Here's how the part is built. I have some questions about the finished solid (model axes, mm). Face numbers are marked on the shaded views. Give positions to 0.01 mm unless a question says otherwise; leave off trailing zeros. Write each loop counter-clockwise with the first axis right and the second up, starting at its lowest first coordinate (ties: lowest second). Pieces come first, ordered by that corner, then holes. Notation, with made-up numbers: (10, -24.5) -> (36, -24.5) arc R37 cw to (36, 11.5) -> close; hole circle Ø4 at (81, 33). An arc over 180 degrees is marked (long way). Use one line per item in the form item = value.
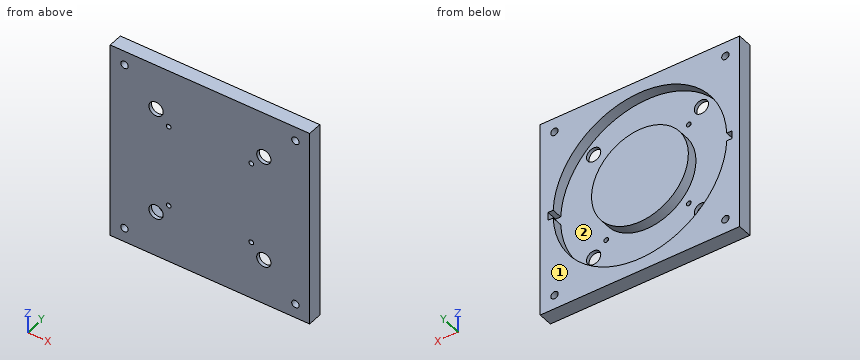
```python
from build123d import *

# Parameters (mm, degrees)
SKETCH_1_W          = 140
SKETCH_1_H          = 140
SKETCH_1_R          = 5
SKETCH_1_R_2        = 1.65
EXTRUDE_1_DEPTH     = 10
SKETCH_2_R          = 2.6
CUT_EXTRUDE_1_DEPTH = 100.498743711
SKETCH_3_R          = 61
SKETCH_3_R_2        = 46
CUT_EXTRUDE_2_DEPTH = 7.5
SKETCH_4_R          = 46
SKETCH_4_R_2        = 34
CUT_EXTRUDE_3_DEPTH = 7.5
SKETCH_5_W          = 7
SKETCH_5_H          = 5.7
CUT_EXTRUDE_4_DEPTH = 7.5


with BuildPart() as part:
    # 草图1 → 凸台-拉伸1 (new body)
    with BuildSketch(Plane(origin=(0, 0, 0), x_dir=(1, 0, 0), z_dir=(0, 1, 0))):
        Rectangle(SKETCH_1_W, SKETCH_1_H)
        with Locations(Location((-37.830212793, 37.830212793, 0), (0, 0, 270))):
            Circle(SKETCH_1_R, mode=Mode.SUBTRACT)
        with Locations(Location((-28.991378029, 28.991378029, 0), (0, 0, 270))):
            Circle(SKETCH_1_R_2, mode=Mode.SUBTRACT)
        with Locations(Location((28.991378029, 28.991378029, 0), (0, 0, 270))):
            Circle(SKETCH_1_R_2, mode=Mode.SUBTRACT)
        with Locations(Location((37.830212793, 37.830212793, 0), (0, 0, 270))):
            Circle(SKETCH_1_R, mode=Mode.SUBTRACT)
        with Locations(Location((28.991378029, -28.991378029, 0), (0, 0, 270))):
            Circle(SKETCH_1_R_2, mode=Mode.SUBTRACT)
        with Locations(Location((37.830212793, -37.830212793, 0), (0, 0, 270))):
            Circle(SKETCH_1_R, mode=Mode.SUBTRACT)
        with Locations(Location((-28.991378029, -28.991378029, 0), (0, 0, 270))):
            Circle(SKETCH_1_R_2, mode=Mode.SUBTRACT)
        with Locations(Location((-37.830212793, -37.830212793, 0), (0, 0, 270))):
            Circle(SKETCH_1_R, mode=Mode.SUBTRACT)
    extrude(amount=EXTRUDE_1_DEPTH)

    # 草图2 → 切除-拉伸1 (cut, through all)
    with BuildSketch(Plane(origin=(0, 10, 0), x_dir=(1, 0, 0), z_dir=(0, 1, 0))):
        with Locations(Location((-60, 60, 0), (0, 0, 270))):
            Circle(SKETCH_2_R)
        with Locations(Location((60, 60, 0), (0, 0, 270))):
            Circle(SKETCH_2_R)
        with Locations(Location((60, -60, 0), (0, 0, 270))):
            Circle(SKETCH_2_R)
        with Locations(Location((-60, -60, 0), (0, 0, 270))):
            Circle(SKETCH_2_R)
    extrude(amount=-CUT_EXTRUDE_1_DEPTH, mode=Mode.SUBTRACT)

    # 草图3 → 切除-拉伸2 (cut)
    with BuildSketch(Plane(origin=(0, 10, 0), x_dir=(1, 0, 0), z_dir=(0, 1, 0))):
        with Locations(Location((0, 0, 0), (0, 0, 270))):
            Circle(SKETCH_3_R)
        with Locations(Location((0, 0, 0), (0, 0, 270))):
            Circle(SKETCH_3_R_2, mode=Mode.SUBTRACT)
    extrude(amount=-CUT_EXTRUDE_2_DEPTH, mode=Mode.SUBTRACT)

    # 草图4 → 切除-拉伸3 (cut)
    with BuildSketch(Plane(origin=(0, 10, 0), x_dir=(1, 0, 0), z_dir=(0, 1, 0))):
        Circle(SKETCH_4_R)
        with Locations(Location((0, 0, 0), (0, 0, 270))):
            Circle(SKETCH_4_R_2, mode=Mode.SUBTRACT)
    extrude(amount=-CUT_EXTRUDE_3_DEPTH, mode=Mode.SUBTRACT)

    # 草图5 → 切除-拉伸4 (cut)
    with BuildSketch(Plane(origin=(0, 10, 0), x_dir=(1, 0, 0), z_dir=(0, 1, 0))):
        with Locations((-61, 0)):
            Rectangle(SKETCH_5_W, SKETCH_5_H)
        with Locations((61, 0)):
            Rectangle(SKETCH_5_W, SKETCH_5_H)
    extrude(amount=-CUT_EXTRUDE_4_DEPTH, mode=Mode.SUBTRACT)


solid = part.part
```
Q1. If we mould it in two halves opening along X, with no side actions, what happens to the marked faces 1 and 2? For each: +X half, -X half, draft (parallel to the pull), parting line (faces both ways), or undercut.
Result set:
face_1 = draft
face_2 = undercut
Q2. If I drill on line 1 along X through (y, z) = (8, -17.5); line 2 along Z through (x, y) = (-37, 2); line 3 along X through (y, z) = (7.75, 19), over which ranges is the centre line in solid material (lowest first)? Write a range as from..to.
Result set:
line_1 = -70..-58.44, -29.15..29.15, 58.44..70
line_2 = -70..-42.76, -32.9..32.9, 42.76..70
line_3 = -70..-57.97, -28.2..28.2, 57.97..70
Q3. I want a section at A-A, the plane y = 8.5. Write out the boundary of the cut face in (x, z).
Result set:
outline = (-70, -70) -> (70, -70) -> (70, 70) -> (-70, 70) -> close; circle Ø68 at (0, 0); hole (-64.5, -2.85) -> (-60.93, -2.85) arc R61 ccw to (60.93, -2.85) -> (64.5, -2.85) -> (64.5, 2.85) -> (60.93, 2.85) arc R61 ccw to (-60.93, 2.85) -> (-64.5, 2.85) -> close; hole circle Ø5.2 at (-60, -60); hole circle Ø5.2 at (-60, 60); hole circle Ø5.2 at (60, -60); hole circle Ø5.2 at (60, 60)
Q4. Will this pin go through, and if not, where does the flat tip stop? pin 1 Ø1.5 at (x, z) = (-29.5, -30) entering from +Y.
Result set:
pin_1 = 2.5
Q5. I want a section at C-C, the plane z = 49. Write out the boundary of the cut face in (x, y).
Result set:
outline = (-70, 0) -> (70, 0) -> (70, 10) -> (36.33, 10) -> (36.33, 2.5) -> (-36.33, 2.5) -> (-36.33, 10) -> (-70, 10) -> close
Q6. I want a section at B-B, the plane x = 45. Write out the boundary of the cut face in (y, z), and give its area (3 significant figures).
Result set:
outline = (0, -70) -> (10, -70) -> (10, -41.18) -> (2.5, -41.18) -> (2.5, 41.18) -> (10, 41.18) -> (10, 70) -> (0, 70) -> close
area = 782 mm2
Q7. I want a section at D-D, the plane z = 16.5. Write out the boundary of the cut face in (x, y), and give its area (3 significant figures).
Result set:
outline = (-70, 0) -> (70, 0) -> (70, 10) -> (58.73, 10) -> (58.73, 2.5) -> (29.73, 2.5) -> (29.73, 10) -> (-29.73, 10) -> (-29.73, 2.5) -> (-58.73, 2.5) -> (-58.73, 10) -> (-70, 10) -> close
area = 965 mm2
